```python
from build123d import *

# Parameters (mm, degrees)
ANGLES_EQUAL_90_X_90_X_8_1_DEPTH = 180
SKETCH12_R                       = 13
CUT_EXTRUDE1_DEPTH               = 221.45407685
LPATTERN1_COUNT                  = 2
LPATTERN1_PITCH                  = 90
CUT_EXTRUDE2_REACH               = 219.311
SKETCH13_R                       = 13
LPATTERN2_COUNT                  = 2
LPATTERN2_PITCH                  = 90


with BuildPart() as part:
    # Sketch11 → Angles equal 90 X 90 X 8(1) (new body)
    with BuildSketch(Plane(origin=(0, 45, 45), x_dir=(0, 1, 0), z_dir=(1, 0, 0))):
        with BuildLine():
            Line((-45, 45), (-45, -45))
            Line((-45, -45), (45, -45))
            Line((45, -45), (45, -42.5))
            ThreePointArc((45, -42.5), (43.389087297, -38.610912703), (39.5, -37))
            Line((39.5, -37), (-26, -37))
            ThreePointArc((-26, -37), (-33.778174593, -33.778174593), (-37, -26))
            Line((-37, -26), (-37, 39.5))
            ThreePointArc((-37, 39.5), (-38.610912703, 43.389087297), (-42.5, 45))
            Line((-42.5, 45), (-45, 45))
        make_face()
    extrude(amount=ANGLES_EQUAL_90_X_90_X_8_1_DEPTH)

    # Sketch12 → Cut-Extrude1 (cut, symmetric)
    with BuildSketch(Plane(origin=(0, 0, 0), x_dir=(1, 0, 0), z_dir=(0, 1, 0))):
        with Locations(Location((45, -55, 0), (0, 0, 90))):
            Circle(SKETCH12_R)
    cut_extrude1 = extrude(amount=CUT_EXTRUDE1_DEPTH, both=True, mode=Mode.SUBTRACT)

    # LPattern1: Cut-Extrude1 ×2
    with Locations(*[(i * LPATTERN1_PITCH, 0, 0) for i in range(1, LPATTERN1_COUNT)]):
        add(cut_extrude1, mode=Mode.SUBTRACT)

    # Sketch13 → Cut-Extrude2 (cut, up to next)
    with BuildSketch(Plane.XY.offset(8), mode=Mode.PRIVATE) as cut_extrude2_sk1:
        with Locations((45, 55)):
            Circle(SKETCH13_R)
    cut_extrude2_tool1 = extrude(cut_extrude2_sk1.sketch, amount=-CUT_EXTRUDE2_REACH, mode=Mode.PRIVATE) & part.part
    cut_extrude2 = cut_extrude2_tool1.solids().sort_by_distance((45, 55, 8))[0]
    add(cut_extrude2, mode=Mode.SUBTRACT)

    # LPattern2: Cut-Extrude2 ×2
    with Locations(*[(i * LPATTERN2_PITCH, 0, 0) for i in range(1, LPATTERN2_COUNT)]):
        add(cut_extrude2, mode=Mode.SUBTRACT)


solid = part.part
```
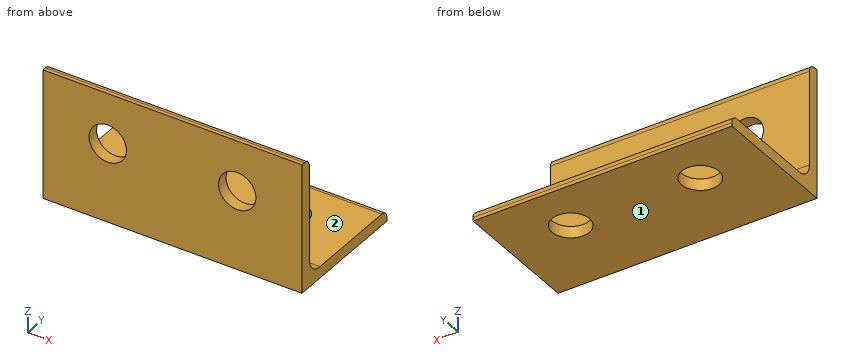
Build history of the part. All positions in model axes, mm. Face numbers are marked on the shaded views. A direction names the side the tool comes from. Give positions to 0.01 mm unless a question says otherwise; leave off trailing zeros. Order: outer loops, then holes, each group sorted by start corner. A loop starts at its lowest first (then second) coordinate and runs counter-clockwise, first axis right, second up. Notation, with made-up numbers: M 58.5,40 L 74.5,40 A23 cw 74.5,75 Z; hole C 42,-15 d10. An arc over 180 degrees is marked long. Return JSON: item names as keys, results as strings.
Q1. 3-axis set-ups, long thin cutter, end or side, ignore diameter. For the marked faces 1 and 2: which of +Z, -Z, +X, -X, +Y, -Y reach the whole face in a straight line?
Answer list:
{"face 1": "-Z, +X, -X, +Y, -Y", "face 2": "+Z, +X, -X, +Y"}
Q2. Flat gauge pins, fed straight in: pin 1 (15.5 mm diameter, centred on x = 45, z = 55, fed in from -Y); pin 2 (10 mm diameter, centred on x = 34.5, y = 80, fed in from +Z); pin 3 (8 mm diameter, centred on x = 29, z = 81, fed in from +Y). Where does each tip first touch, or does it go through?
Answer list:
{"pin 1": "passes through", "pin 2": "stops at z = 8", "pin 3": "stops at y = 8"}
Q3. Band-saw the part on B-B (x = 135). Give the cut face in (y, z).
Answer list:
{"outline": "M 0,0 L 42,0 L 42,8 L 19,8 A11 cw 8,19 L 8,42 L 0,42 Z; M 0,68 L 8,68 L 8,84.5 A5.5 ccw 2.5,90 L 0,90 Z; M 68,0 L 90,0 L 90,2.5 A5.5 ccw 84.5,8 L 68,8 Z"}
Q4. Wall check: probe 1 along X at (y, z) = (2, 55); probe 2 along Z at (x, y) = (45, 3); probe 3 along Z at (x, y) = (125, 39). Give the ranges that are in metal, low to high. Write a range as from..to.
Answer list:
{"probe 1": "x = 0..32, 58..122, 148..180", "probe 2": "z = 0..42, 68..89.98", "probe 3": "z = 0..8"}
Q5. Band-saw the part on D-D (x = 75). Give the cut face in (y, z), then the cut area to 3 significant figures.
Answer list:
{"outline": "M 0,0 L 90,0 L 90,2.5 A5.5 ccw 84.5,8 L 19,8 A11 cw 8,19 L 8,84.5 A5.5 ccw 2.5,90 L 0,90 Z", "area": "1,390 mm^2"}
Q6. Band-saw the part on A-A (y = 55). Give the cut face in (x, z), then the cut area to 3 significant figures.
Answer list:
{"outline": "M 0,0 L 32,0 L 32,8 L 0,8 Z; M 58,0 L 122,0 L 122,8 L 58,8 Z; M 148,0 L 180,0 L 180,8 L 148,8 Z", "area": "1,020 mm^2"}
